from build123d import *

# Parameters (mm, degrees)
F0_W        = 117
F0_H        = 154.5
F0_H_2      = 150.5
F0_W_2      = 67.4791876724
F2_R        = 1.5875
F3_SIZE     = 0.7696969697
F4_C1_SIZE2 = 6.35
F4_C1_SIZE  = 16.51
F4_C2_SIZE2 = 16.51
F4_C2_SIZE  = 6.35


with BuildPart() as f1:
    # F0 (on Right) → F1 (revolve)
    with BuildSketch(Plane.YZ):
        with Locations((58.5, 267.75)):
            Rectangle(F0_W, F0_H)
        with Locations((58.5, 115.25)):
            Rectangle(F0_W, F0_H_2)
        with Locations((150.7395938362, 115.25)):
            Rectangle(F0_W_2, F0_H_2)
    revolve(axis=Axis((0, 115.410885826, 0), (0, 1, 0)))

    # F2
    f2_edges = [f1.edges().sort_by_distance(p)[0] for p in [
        (0, 117, -190.5),
    ]]
    fillet(f2_edges, radius=F2_R)

    # F3
    f3_edges = [f1.edges().sort_by_distance(p)[0] for p in [
        (0, 184.479188, -190.5),
    ]]
    chamfer(f3_edges, length=F3_SIZE)

    # F4: chamfer of 6.35 x 16.51 on 4 edges, made by hand

    # F4_c1
    f4_c1_edges = [f1.edges().sort_by_distance(p)[0] for p in [
        (0, 117, -345),
    ]]
    f4_c1_side = f1.faces().sort_by_distance((0, 117, -344.873))[0]
    chamfer(f4_c1_edges, length=F4_C1_SIZE, length2=F4_C1_SIZE2, reference=f4_c1_side)

    # F4_c2
    f4_c2_edges = [f1.edges().sort_by_distance(p)[0] for p in [
        (0, 0, -345),
    ]]
    f4_c2_side = f1.faces().sort_by_distance((0, 0.127, -345))[0]
    chamfer(f4_c2_edges, length=F4_C2_SIZE, length2=F4_C2_SIZE2, reference=f4_c2_side)


solid = f1.part
Source: CAD feature listing. Evaluate the final solid. Frame: model axes, mm. A direction names the side the tool comes from. Coordinates: 2 decimals unless noted, no trailing zeros. Order: outer loops, then holes, each group sorted by start corner. A loop starts at its lowest first (then second) coordinate and runs counter-clockwise, first axis right, second up. Notation, with made-up numbers: M 32,-17 L 78,-17 A29 ccw 78,7 Z; hole C 46,-30.5 d8. An arc over 180 degrees is marked long. Write each question's results on one line, items separated by ' | '. Start each with the question number.
1. Section C-C, the plane y = 97. Return the cut outline in (x, z), then the cut area to 3 significant figures.
2. Pin query (flat end, axial travel): pin 1 (8 mm diameter, centred on y = 86.5, z = 219, fed in from +X); pin 2 (1.5 mm diameter, centred on x = 174.5, y = 98.5, fed in from +Z); pin 3 (4 mm diameter, centred on y = 82.5, z = 62, fed in from +X); pin 4 (6 mm diameter, centred on x = -64.5, z = 149.5, fed in from -Y). Return the tip coordinate at first contact, or that it passes through.
3. Reachability of faces 4 (the face through (-115.92, 151.6, -151.17)), 5 (the face through (-321.461, 0.308, -71.384)) from +Z, -Z, +X, -X, +Y, -Y: full face, straight path, thin tool, end or side. Return the list, or none.
4. Draft query along Z for faces 1 (the face through (103.63, 59.23, 329.07)), 2 (the face through (-39.05, 93.53, -8.67)), 3 (the face through (-141, 117, -141)). Return one class per face: +Z half, -Z half, draft (parallel to the pull), parting line (faces both ways), or undercut.
5. Material intervals for L1, parallel to X at y = 90, z = 0; L2, parallel to X at y = 146, z = 0; L3, parallel to Y at x = 126, z = 196, sorted ascending.
Solution:
1) outline: C 0,0 d690; hole C 0,0 d80 | area: 369,000 mm²
2) pin 1: x = 269.81 | pin 2: z = 298.05 | pin 3: x = 339.74 | pin 4: y = 0
3) face 4: +Y | face 5: -Y
4) face 1: parting line | face 2: undercut | face 3: draft
5) L1: -345 to -40, 40 to 345 | L2: -190.5 to -40, 40 to 190.5 | L3: 0 to 117
